Part model, mm, in its own coordinate system. A direction names the side the tool comes from. Coordinates: 2 decimals unless noted, no trailing zeros. Loops run counter-clockwise (first coordinate to the right, second up) from the corner with the lowest first, then second, coordinate; pieces in that order, holes last. Notation, with made-up numbers: (-21.75, -12) - (-15.75, -12) arc R22 cw to (-15.75, 2) - close; hole circle Ø7 at (78, 0). An arc over 180 degrees is marked (long way). Use a Markdown table: item, result. Add a question column.
1. Pull direction Y, two halves, no side cores. Call faces 1 (the flat face through (0, 8, 1)), 2 (the flat face through (-6, -24, 3)), 3 (the flat face through (-0.1, -50, 0.6)): pulls with the +Y half, pulls with the -Y half, needs draft (parallel to the pull), parting line crosses it, or undercut.
2. Band-saw the part on B-B, the plane z = 2.25. Give the cut face in (x, y), plus the area to 3 significant figures.
3. Drop flat-ended pins along their axis: pin 1 (8 mm diameter, centred on x = 14, y = 13.5, fed in from +Z); pin 2 (10 mm diameter, centred on x = -19, y = -4.5, fed in from -Z); pin 3 (0.9 mm diameter, centred on y = -25, z = 2, fed in from +X); pin 4 (1.5 mm diameter, centred on x = 16.5, z = 1.5, fed in from -Y). Give the stop position or say it passes through.
4. Band-saw the part on C-C, the plane x = -22.5. Give the cut face in (y, z).
5. Band-saw the part on A-A, the plane y = -8.5. Give the cut face in (x, z).
6. 3-axis set-ups, long thin cutter, end or side, ignore diameter. For faces 4 (the flat face through (6, -25, 3)), 5 (the cylindrical face through (-29, 15, 3)), 6 (the flat face through (-7, -25, 2)), 7 (the flat face through (7, -25, 2)): which of +Z, -Z, +X, -X, +Y, -Y reach the whole face in a straight line?
7. Wall check: probe 1 along X at (y, z) = (-11, 3.2); probe 2 along Z at (x, y) = (0, -30.5); probe 3 along Y at (x, z) = (-14, 3.15). Give the ranges that are in metal, low to high. Write a range as [from, to].
from build123d import *

# Parameters (mm, degrees)
PAD_DEPTH    = 4
POCKET_DEPTH = 3


with BuildPart() as part:
    # Sketch → Pad (new body)
    with BuildSketch(Plane.XY):
        with BuildLine():
            Line((-7, -50), (7, -50))
            Line((7, -50), (7, 0))
            Line((7, 0), (15, 0))
            ThreePointArc((15, 0), (30, 15), (15, 30))
            Line((15, 30), (-15, 30))
            ThreePointArc((-15, 30), (-30, 15), (-15, 0))
            Line((-15, 0), (-7, 0))
            Line((-7, 0), (-7, -50))
        make_face()
    extrude(amount=PAD_DEPTH)

    # Sketch001 → Pocket (cut)
    with BuildSketch(Plane.XY.offset(4)):
        with BuildLine():
            Line((-6, -50), (6, -50))
            Line((6, -50), (6, 1))
            Line((6, 1), (15, 1))
            ThreePointArc((15, 1), (29, 15), (15, 29))
            Line((15, 29), (-15, 29))
            ThreePointArc((-15, 29), (-29, 15), (-15, 1))
            Line((-15, 1), (-6, 1))
            Line((-6, 1), (-6, -50))
        make_face()
    extrude(amount=-POCKET_DEPTH, mode=Mode.SUBTRACT)


solid = part.part
Geometry check:
| question | item | result |
|---|---|---|
| 1 | face 1 | undercut |
| 1 | face 2 | needs draft |
| 1 | face 3 | pulls with the -Y half |
| 2 | outline | (-15, 0) - (-7, 0) - (-7, -50) - (-6, -50) - (-6, 1) - (-15, 1) arc R14 cw to (-15, 29) - (15, 29) arc R14 cw to (15, 1) - (6, 1) - (6, -50) - (7, -50) - (7, 0) - (15, 0) arc R15 ccw to (15, 30) - (-15, 30) arc R15 ccw to start |
| 2 | area | 239 mm^2 |
| 3 | pin 1 | stops at z = 1 |
| 3 | pin 2 | stops at z = 0 |
| 3 | pin 3 | stops at x = 7 |
| 3 | pin 4 | stops at y = 0.02 |
| 4 | outline | (2.01, 0) - (27.99, 0) - (27.99, 4) - (26.82, 4) - (26.82, 1) - (3.18, 1) - (3.18, 4) - (2.01, 4) - close |
| 5 | outline | (-7, 0) - (7, 0) - (7, 4) - (6, 4) - (6, 1) - (-6, 1) - (-6, 4) - (-7, 4) - close |
| 6 | face 4 | +Z, -Y |
| 6 | face 5 | +Z |
| 6 | face 6 | +Z, -Z, -X, -Y |
| 6 | face 7 | +Z, -Z, +X, -Y |
| 7 | probe 1 | x = [-7, -6], [6, 7] |
| 7 | probe 2 | z = [0, 1] |
| 7 | probe 3 | y = [0, 1], [29, 30] |
